Geometry: final body of the model. Coordinates: model frame, mm. A direction names the side the tool comes from. Give positions to 0.01 mm unless a question says otherwise; leave off trailing zeros. Loops run counter-clockwise (first coordinate to the right, second up) from the corner with the lowest first, then second, coordinate; pieces in that order, holes last.
from build123d import *

# Parameters (mm, degrees)
BOSS_EXTRUDE1_DEPTH = 12
CUT_EXTRUDE1_DEPTH  = 10.6
SKETCH3_R           = 0.8
CUT_EXTRUDE2_DEPTH  = 16.274572476
SKETCH4_R           = 1.025
CUT_EXTRUDE3_DEPTH  = 6
FILLET1_R           = 6
FILLET2_R           = 2
CUT_EXTRUDE4_DEPTH  = 1.2
FILLET3_R           = 2
SKETCH6_W           = 8
SKETCH6_H           = 3
BOSS_EXTRUDE2_DEPTH = 10


# Some blends are built 0.0001 mm under size
with BuildPart() as part:
    # Sketch1 → Boss-Extrude1 (new body)
    with BuildSketch(Plane(origin=(0, 0, 0), x_dir=(1, 0, 0), z_dir=(0, 1, 0))):
        Polygon((-16.635707691, 24.623874564), (7.964292309, 24.623874564), (7.964292309, -24.376125436), (-5.235707691, -24.376125436), (-5.235707691, 10.623874564), (-12.635707691, 10.623874564), (-12.635707691, -4.376125436), (-16.635707691, -4.376125436), align=None)
    extrude(amount=BOSS_EXTRUDE1_DEPTH)

    # Sketch2 → Cut-Extrude1 (cut)
    with BuildSketch(Plane(origin=(0, 12, 0), x_dir=(1, 0, 0), z_dir=(0, 1, 0))):
        Polygon((-3.435707691, -18.376125436), (6.764292309, -18.376125436), (6.764292309, 18.623874564), (-15.635707691, 18.623874564), (-15.635707691, 11.89844704), (-3.435707691, 11.89844704), align=None)
    extrude(amount=-CUT_EXTRUDE1_DEPTH, mode=Mode.SUBTRACT)

    # Sketch3 → Cut-Extrude2 (cut)
    with BuildSketch(Plane.XY.offset(4.376125436)):
        with Locations((-14.635707691, 12)):
            Circle(SKETCH3_R)
    extrude(amount=-CUT_EXTRUDE2_DEPTH, mode=Mode.SUBTRACT)

    # Sketch4 → Cut-Extrude3 (cut)
    with BuildSketch(Plane(origin=(0, 12, 0), x_dir=(1, 0, 0), z_dir=(0, 1, 0))):
        with Locations(Location((-10.035707691, 21.623874564, 0), (0, 0, 270))):
            Circle(SKETCH4_R)
        with Locations(Location((1.364292309, 21.623874564, 0), (0, 0, 270))):
            Circle(SKETCH4_R)
        with Locations(Location((1.364292309, -21.376125436, 0), (0, 0, 270))):
            Circle(SKETCH4_R)
    extrude(amount=-CUT_EXTRUDE3_DEPTH, mode=Mode.SUBTRACT)

    # Fillet1
    fillet1_edges = [part.edges().sort_by_distance(p)[0] for p in [
        (-16.635707691, 6, -24.623874564),
        (7.964292309, 6, -24.623874564),
        (7.964292309, 6, 24.376125436),
        (-5.235707691, 6, 24.376125436),
    ]]
    fillet(fillet1_edges, radius=FILLET1_R)

    # Fillet2
    fillet2_edges = [part.edges().sort_by_distance(p)[0] for p in [
        (-5.235707691, 6, -10.623874564),
        (-12.635707691, 6, -10.623874564),
        (-12.635707691, 6, 4.376125436),
        (-16.635707691, 6, 4.376125436),
    ]]
    fillet(fillet2_edges, radius=FILLET2_R - 0.0001)  # a hair under: the kernel refuses the full size

    # Sketch5 → Cut-Extrude4 (cut)
    with BuildSketch(Plane(origin=(7.964292309, 0, 0), x_dir=(0, 0, -1), z_dir=(1, 0, 0))):
        with BuildLine():
            Line((-3.376125436, 8.6), (-3.376125436, 12))
            Line((-3.376125436, 12), (1.023874564, 12))
            Line((1.023874564, 12), (1.023874564, 8.6))
            ThreePointArc((1.023874564, 8.6), (-1.176125436, 6.4), (-3.376125436, 8.6))
        make_face()
    extrude(amount=-CUT_EXTRUDE4_DEPTH, mode=Mode.SUBTRACT)

    # Fillet3
    # the kernel refuses this fillet: 2 mm, written as the material it takes off along each edge
    with BuildSketch(Plane(origin=(-3.435707691, 17, -11.89844704), x_dir=(-1, 0, 0), z_dir=(0, -1, 0))) as fillet3_piece_1:
        with BuildLine():
            CenterArc((FILLET3_R, -FILLET3_R), FILLET3_R, 90, 90)
            Line((0, -FILLET3_R), (0, 0))
            Line((0, 0), (FILLET3_R, 0))
        make_face()
    extrude(amount=15.6, mode=Mode.SUBTRACT)
    with BuildSketch(Plane(origin=(-14.635707691, 12, -11.89844704), x_dir=(-0.0031415874858797778, 0.9999950652018582, 0), z_dir=(0.9999950652018582, 0.0031415874858797778, 0))) as fillet3_piece_2_section:
        with BuildLine():
            CenterArc((0.8 + FILLET3_R, 0 + FILLET3_R), FILLET3_R, 180, 90)
            Line((0.8 + FILLET3_R, 0), (0.8, 0))
            Line((0.8, 0), (0.8, 0 + FILLET3_R))
        make_face()
    fillet3_piece_2 = revolve(axis=Axis((-14.635707691, 12, -11.89844704), (0, 0, 1)), revolution_arc=359.64, mode=Mode.PRIVATE)
    fillet3_piece_2 = split(fillet3_piece_2, bisect_by=Plane(origin=(-15.635707691, 11.089592245, -11.483446459), z_dir=(1, 0, 0)), keep=Keep.TOP, mode=Mode.PRIVATE)
    add(fillet3_piece_2, mode=Mode.SUBTRACT)

    # Sketch6 → Boss-Extrude2 (add)
    with BuildSketch(Plane(origin=(0, 1.4, 0), x_dir=(1, 0, 0), z_dir=(0, 1, 0))):
        with Locations((2.764292309, 17.123874564)):
            Rectangle(SKETCH6_W, SKETCH6_H)
    extrude(amount=BOSS_EXTRUDE2_DEPTH)


solid = part.part
Item 1: Draft query along X for faces 1 (the face through (-1, 0, -6)), 2 (the face through (2, 7, 18.376)), 3 (the face through (6.253, 6.084, 22.572)). Return one class per face: +X half, -X half, draft (parallel to the pull), parting line (faces both ways), or undercut.
Values follow:
face 1: draft
face 2: undercut
face 3: +X half
Item 2: Section query D-D on x = -6. Return loops of the section in (y, z), plus the area to 3 significant figures.
Values follow:
outline: (0, -24.62) - (12, -24.62) - (12, -18.62) - (1.4, -18.62) - (1.4, -11.9) - (12, -11.9) - (12, -10.2) - (0, -10.2) - close
area: 102 mm2
Item 3: Section query C-C on z = -17.5. Return loops of the section in (x, y).
Values follow:
outline: (-16.64, 0) - (7.96, 0) - (7.96, 12) - (6.76, 12) - (6.76, 11.4) - (-1.24, 11.4) - (-1.24, 1.4) - (-15.64, 1.4) - (-15.64, 12) - (-16.64, 12) - close
Item 4: Set-up query: faces 4 (the face through (7, 10, -1.024)), 5 (the face through (-4.04, 6.77, -11.33)), 6 (the face through (-12.636, 6, -3)), 7 (the face through (-14.65, 11.2, -2.66)). Return all of +Z, -Z, +X, -X, +Y, -Y with unobstructed straight access to the full face (end or side cutting, diameter ignored); none if empty.
Values follow:
face 4: +X, +Y
face 5: +Y
face 6: +Z, +Y, -Y
face 7: +Z, +Y
Item 5: Pin query (flat end, axial travel): pin 1 (2.5 mm diameter, centred on x = 2, z = -22, fed in from +Y); pin 2 (1 mm diameter, centred on x = -9.5, z = -13.5, fed in from +Y); pin 3 (1.3 mm diameter, centred on x = 7.5, y = 10, fed in from -Z); pin 4 (2.5 mm diameter, centred on x = -8.5, y = 8.5, fed in from +Z). Return the tip coordinate at first contact, or that it passes through.
Values follow:
pin 1: stops at y = 12
pin 2: stops at y = 1.4
pin 3: stops at z = -22.11
pin 4: stops at z = -10.62
Item 6: Section query A-A on z = -5. Return loops of the section in (x, y).
Values follow:
outline: (-16.64, 0) - (-12.64, 0) - (-12.64, 12) - (-13.84, 12) arc R0.8 cw to (-15.44, 12) - (-16.64, 12) - close; (-5.24, 0) - (7.96, 0) - (7.96, 12) - (6.76, 12) - (6.76, 1.4) - (-3.44, 1.4) - (-3.44, 12) - (-5.24, 12) - close
Item 7: Ray query, probe 1 along X at (y, z) = (1.5, -4); probe 2 along X at (y, z) = (7.5, -16.5); probe 3 along X at (y, z) = (11.5, -6). Return the intervals inside material, ascending.
Values follow:
probe 1: x = -16.64 to -12.64, -5.24 to -3.44, 6.76 to 7.96
probe 2: x = -16.64 to -15.64, -1.24 to 7.96
probe 3: x = -16.64 to -15.26, -14.01 to -12.64, -5.24 to -3.44, 6.76 to 7.96
